Autodesk Fusion 360 part; units mm, degrees
sketch "Sketch1" plane through (0, 0, 0) normal (0, 1, 0) x (1, 0, 0)
  line L0 (0, 0) -> (18.4, 0)
  line L1 (18.4, 0) -> (18.4, -34)
  line L2 (18.4, -34) -> (0, -34)
  line L3 (0, -34) -> (0, 0)
  circle A0 centre (9.2, -24.8) radius 9.2
  circle A1 centre (9.2, -24.8) radius 4.3
  dimension "d1" = 18.4
  dimension "d2" = 34
  dimension "d3" = 4.9
extrude "Extrude2" add sketch "Sketch1" along normal blind 18 contours L0 L1 L3 A0 | A0
fillet "Fillet1" radius 0.5 6 edges at (18.4, 0, 12.4) (9.2, 0, 34) (0, 0, 12.4) (0, 18, 12.4) (9.2, 18, 34) (18.4, 18, 12.4)
sketch "Sketch2" plane through (0, 0, 0) normal (0, 0, 1) x (1, 0, 0)
  line L0 (18.4, 0.5) -> (18.4, 17.5)
sketch "Sketch3" plane through (0, 0, 0) normal (0, 0, 1) x (1, 0, 0)
  circle A0 centre (9.2, 9.2591) radius 2.3
  dimension "d9" = 4.6
extrude "Extrude3" cut sketch "Sketch3" along normal blind 17
Build history of the part. All positions in model axes, mm. Round coordinates to 2 decimals unless told otherwise and drop trailing zeros. Order: outer loops, then holes, each group sorted by start corner. A loop starts at its lowest first (then second) coordinate and runs counter-clockwise, first axis right, second up. Notation, with made-up numbers: (86, 89) -> (105, 89) arc R30 cw to (105, 115) -> close; hole circle Ø8 at (-14, 30). An arc over 180 degrees is marked (long way). Answer in a Markdown table with one row per item.
1) Band-saw the part on A-A on x = 9.2. Give the cut face in (y, z), and give its area (3 significant figures).
Values:
| item | result |
|---|---|
| outline | (0, 0) -> (6.96, 0) -> (6.96, 17) -> (11.56, 17) -> (11.56, 0) -> (18, 0) -> (18, 20.5) -> (0, 20.5) -> close; (0, 29.1) -> (18, 29.1) -> (18, 33.5) arc R0.5 ccw to (17.5, 34) -> (0.5, 34) arc R0.5 ccw to (0, 33.5) -> close |
| area | 379 mm2 |
2) Band-saw the part on B-B on y = 2.5. Give the cut face in (x, z), and give its area (3 significant figures).
Values:
| item | result |
|---|---|
| outline | (0, 0) -> (18.4, 0) -> (18.4, 24.8) arc R9.2 ccw to (0, 24.8) -> close; hole circle Ø8.6 at (9.2, 24.8) |
| area | 531 mm2 |
3) Wall check: L1, parallel to X at y = 13.5, z = 24.8; L2, parallel to Y at x = 9.2, z = 13.25; L3, parallel to Z at x = 9.2, y = 11.5. Give the ranges that are in metal, low to high.
Values:
| item | result |
|---|---|
| L1 | 0 to 4.9, 13.5 to 18.4 |
| L2 | 0 to 6.96, 11.56 to 18 |
| L3 | 17 to 20.5, 29.1 to 34 |
4) Mould opens along X. For faces 1 (the cylindrical face through (10.44, 7.32, 8.38)), 2 (the flat face through (9, 9, 17)), 3 (the cylindrical face through (9.402, 8.881, 33.998)), 4 (the flat face through (18.4, 9, 12)) say: released by +X, released by -X, zero draft, split by the parting line, or undercut.
Values:
| item | result |
|---|---|
| face 1 | undercut |
| face 2 | undercut |
| face 3 | split by the parting line |
| face 4 | released by +X |
5) Band-saw the part on C-C on z = 10. Give the cut face in (x, y).
Values:
| item | result |
|---|---|
| outline | (0, 0.5) arc R0.5 ccw to (0.5, 0) -> (17.9, 0) arc R0.5 ccw to (18.4, 0.5) -> (18.4, 17.5) arc R0.5 ccw to (17.9, 18) -> (0.5, 18) arc R0.5 ccw to (0, 17.5) -> close; hole circle Ø4.6 at (9.2, 9.26) |
6) Pin check, flat tips, straight feed: P1, Ø2, axis at x = 15, y = 8.5, coming from the +Z side; P2, Ø4, axis at x = 15.5, y = 7.5, coming from the +Z side; P3, Ø1, axis at x = 7.5, y = 10.5, coming from the +Z side; P4, Ø7.5, axis at x = 9.2, z = 24.8, coming from the -Y side. Stop position of each tip, or through.
Values:
| item | result |
|---|---|
| P1 | z = 32.65 |
| P2 | z = 32.93 |
| P3 | z = 33.92 |
| P4 | through |
